from build123d import *

# Parameters (mm, degrees)
SKETCH1_W                   = 3
SKETCH1_H                   = 8
SKETCH1_W_2                 = 30
BOSS_EXTRUDE3_DEPTH         = 3
SKETCH6_W                   = 3
SKETCH6_H                   = 8
BOSS_EXTRUDE5_DEPTH         = 9
FILLET3_RADIUS              = 4
FILLET3_LENGTH              = 3
SKETCH7_R                   = 2
CUT_EXTRUDE1_DEPTH          = 33.748571352
FILLET3_OF_MIRROR1_2_RADIUS = 4
FILLET3_OF_MIRROR1_2_LENGTH = 3


with BuildPart() as part:
    # Sketch1 → Boss-Extrude3 (new body)
    with BuildSketch(Plane.XY):
        with Locations((-35.895657312, 1.33562795)):
            Rectangle(SKETCH1_W, SKETCH1_H)
        with Locations((-19.395657312, 1.33562795)):
            Rectangle(SKETCH1_W_2, SKETCH1_H)
    boss_extrude3 = extrude(amount=BOSS_EXTRUDE3_DEPTH)

    # Sketch6 → Boss-Extrude5 (add)
    with BuildSketch(Plane.XY.offset(3)):
        with Locations((-35.895657312, 1.33562795)):
            Rectangle(SKETCH6_W, SKETCH6_H)
    boss_extrude5 = extrude(amount=BOSS_EXTRUDE5_DEPTH)

    # Fillet3: full round fillet: the end face becomes a half cylinder, R = half its width
    fillet3_face = Plane((-35.895657312, 1.33562795, 12), x_dir=(-1, 0, 0), z_dir=(0, 0, 1))  # on the end face: x along it, z out of the body
    fillet3_slab = fillet3_face.offset(-FILLET3_RADIUS / 2) * Box(FILLET3_LENGTH, 2 * FILLET3_RADIUS, FILLET3_RADIUS, mode=Mode.PRIVATE)  # the body's end, R deep
    fillet3_round = Plane((-35.895657312, 1.33562795, 8), x_dir=(0, 0, 1), z_dir=(-1, 0, 0)) * Cylinder(FILLET3_RADIUS, FILLET3_LENGTH, mode=Mode.PRIVATE)  # its axis R under the face
    add(fillet3_slab - fillet3_round, mode=Mode.SUBTRACT)

    # Sketch7 → Cut-Extrude1 (cut, through all)
    with BuildSketch(Plane(origin=(-34.395657312, 0, 0), x_dir=(0, 0, -1), z_dir=(1, 0, 0))):
        with Locations((-8, 1.33562795)):
            Circle(SKETCH7_R)
    cut_extrude1 = extrude(amount=-CUT_EXTRUDE1_DEPTH, mode=Mode.SUBTRACT)

    # Mirror1: Boss-Extrude3, Boss-Extrude5, Cut-Extrude1 across plane
    add(boss_extrude3.mirror(Plane(origin=(-4.395657312, 0, 0), x_dir=(0, 0, 1), z_dir=(1, 0, 0))))
    add(boss_extrude5.mirror(Plane(origin=(-4.395657312, 0, 0), x_dir=(0, 0, 1), z_dir=(1, 0, 0))))
    add(cut_extrude1.mirror(Plane(origin=(-4.395657312, 0, 0), x_dir=(0, 0, 1), z_dir=(1, 0, 0))), mode=Mode.SUBTRACT)

    # Fillet3 of Mirror1 2: full round fillet: the end face becomes a half cylinder, R = half its width
    fillet3_of_mirror1_2_face = Plane((27.104342688, 1.33562795, 12), x_dir=(1, 0, 0), z_dir=(0, 0, 1))  # on the end face: x along it, z out of the body
    fillet3_of_mirror1_2_slab = fillet3_of_mirror1_2_face.offset(-FILLET3_OF_MIRROR1_2_RADIUS / 2) * Box(FILLET3_OF_MIRROR1_2_LENGTH, 2 * FILLET3_OF_MIRROR1_2_RADIUS, FILLET3_OF_MIRROR1_2_RADIUS, mode=Mode.PRIVATE)  # the body's end, R deep
    fillet3_of_mirror1_2_round = Plane((27.104342688, 1.33562795, 8), x_dir=(0, 0, 1), z_dir=(1, 0, 0)) * Cylinder(FILLET3_OF_MIRROR1_2_RADIUS, FILLET3_OF_MIRROR1_2_LENGTH, mode=Mode.PRIVATE)  # its axis R under the face
    add(fillet3_of_mirror1_2_slab - fillet3_of_mirror1_2_round, mode=Mode.SUBTRACT)


solid = part.part
Input: part model. Units: mm. Frame: model coordinates. A direction names the side the tool comes from. Give positions to 0.01 mm unless a question says otherwise; leave off trailing zeros. Loops run counter-clockwise (first coordinate to the right, second up) from the corner with the lowest first, then second, coordinate; pieces in that order, holes last. Notation, with made-up numbers: (-26, 5.25) -> (12, 5.25) arc R14 cw to (12, 31.25) -> close; hole circle Ø11 at (79.5, -27.75). An arc over 180 degrees is marked (long way). Answer as a JSON object with one key per item and string values. Group by question number.
Item 1: Pin query (flat end, axial travel): P1, Ø4, axis at x = -5, y = -0.5, coming from the +Z side. Return the tip coordinate at first contact, or that it passes through.
Item 2: Reachability of faces 1 (the flat face through (-34.396, 1, 5)), 2 (the cylindrical face through (-35.87, 0.12, 9.59)) from +Z, -Z, +X, -X, +Y, -Y: full face, straight path, thin tool, end or side. Return the list, or none.
Item 3: Cut plane C-C, the plane x = -26.5. Return the cut outline in (y, z).
Item 4: Pull-direction query (X, two-part tool) for faces 3 (the flat face through (-4, 1, 3)), 4 (the flat face through (-37.396, 1, 5)), 5 (the cylindrical face through (-35.92, 1.25, 12)), 6 (the flat face through (25.604, 1, 5)); classes: released by +X, released by -X, zero draft, split by the parting line, or undercut.
Item 5: Cut plane D-D, the plane y = 4.75. Return the cut outline in (x, z), and give its area (3 significant figures).
Item 6: Line query: probe 1 along Y at (x, z) = (27.6, 8); probe 2 along X at (y, z) = (2.5, 11.25); probe 3 along Z at (x, y) = (22, 0.75). Output: solid intervals per line, ascending.
Item 7: Cut plane B-B, the plane y = 0.5. Return the cut outline in (x, z), and give its area (3 significant figures).
Item 8: Cut plane A-A, the plane z = 8.75. Return the cut outline in (x, y).
Checks:
{
 "1": {"P1": "stops at z = 3"},
 "2": {"face 1": "+Z, +Y, -Y", "face 2": "+X, -X"},
 "3": {"outline": "(-2.66, 0) -> (5.34, 0) -> (5.34, 3) -> (-2.66, 3) -> close"},
 "4": {"face 3": "undercut", "face 4": "released by -X", "face 5": "zero draft", "face 6": "undercut"},
 "5": {"outline": "(-37.4, 0) -> (28.6, 0) -> (28.6, 10.08) -> (25.6, 10.08) -> (25.6, 3) -> (-34.4, 3) -> (-34.4, 10.08) -> (-37.4, 10.08) -> close", "area": "241 mm²"},
 "6": {"probe 1": "y = -2.66 to -0.66, 3.34 to 5.34", "probe 2": "x = -37.4 to -34.4, 25.6 to 28.6", "probe 3": "z = 0 to 3"},
 "7": {"outline": "(-37.4, 0) -> (28.6, 0) -> (28.6, 6.18) -> (25.6, 6.18) -> (25.6, 3) -> (-34.4, 3) -> (-34.4, 6.18) -> (-37.4, 6.18) -> close; (-37.4, 9.82) -> (-34.4, 9.82) -> (-34.4, 11.91) -> (-37.4, 11.91) -> close; (25.6, 9.82) -> (28.6, 9.82) -> (28.6, 11.91) -> (25.6, 11.91) -> close", "area": "230 mm²"},
 "8": {"outline": "(-37.4, -2.59) -> (-34.4, -2.59) -> (-34.4, -0.52) -> (-37.4, -0.52) -> close; (-37.4, 3.19) -> (-34.4, 3.19) -> (-34.4, 5.26) -> (-37.4, 5.26) -> close; (25.6, -2.59) -> (28.6, -2.59) -> (28.6, -0.52) -> (25.6, -0.52) -> close; (25.6, 3.19) -> (28.6, 3.19) -> (28.6, 5.26) -> (25.6, 5.26) -> close"}
}
